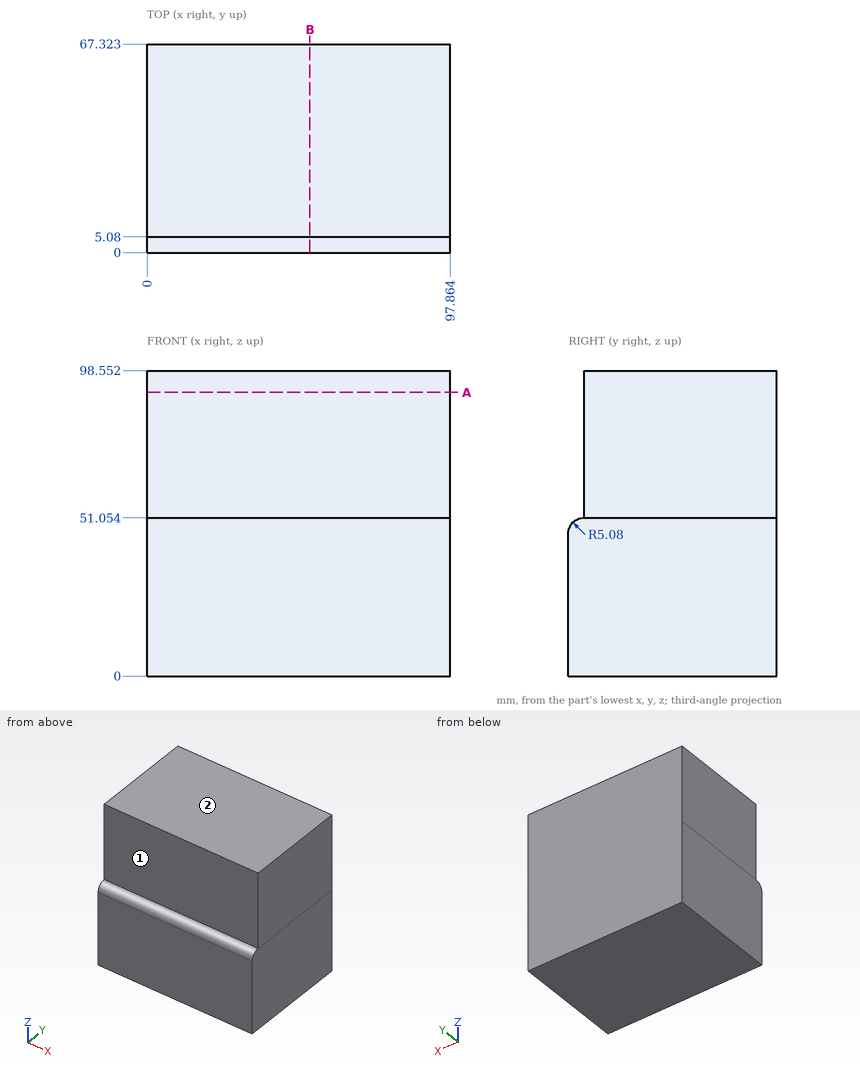
The drawing under review shows one solid part. Ordinate dimensions are in mm from its lowest x, y, z. A direction names the side the tool comes from. Coordinates: 2 decimals unless noted, no trailing zeros. Write each loop counter-clockwise with the first axis right and the second up, starting at its lowest first coordinate (ties: lowest second). Pieces come first, ordered by that corner, then holes. Notation, with made-up numbers: (86.25, 22.25) - (93.25, 22.25) arc R18 ccw to (93.25, 42.25) - close; hole circle Ø8 at (72.25, 27.25). An arc over 180 degrees is marked (long way). Put each result on its own line as item: value.
1. Machinability: for the marked faces 1 and 2, which of the approach directions +Z, -Z, +X, -X, +Y, -Y give a long, thin tool a straight path to every point of the face, cutting with its end or side? Answer none if there is none.
Values found:
face 1: +Z, +X, -X, -Y
face 2: +Z, +X, -X, +Y, -Y
2. Add section A-A, the plane z = 91.5. Give the boundary of the cut face in (x, y), then the cut area to 3 significant figures.
Values found:
outline: (0, 5.08) - (97.86, 5.08) - (97.86, 67.32) - (0, 67.32) - close
area: 6,090 mm²
3. Add section B-B, the plane x = 52.5. Give the boundary of the cut face in (y, z).
Values found:
outline: (0, 0) - (67.32, 0) - (67.32, 98.55) - (5.08, 98.55) - (5.08, 51.05) arc R5.08 ccw to (0, 45.97) - close
4. Wall thickness on probe 1 along Y at (x, z) = (32, 74.5); probe 2 along Z at (x, y) = (92.5, 4): over which ranges is each line inside the solid? List them lowest first.
Values found:
probe 1: 5.08 to 67.32
probe 2: 0 to 50.94
